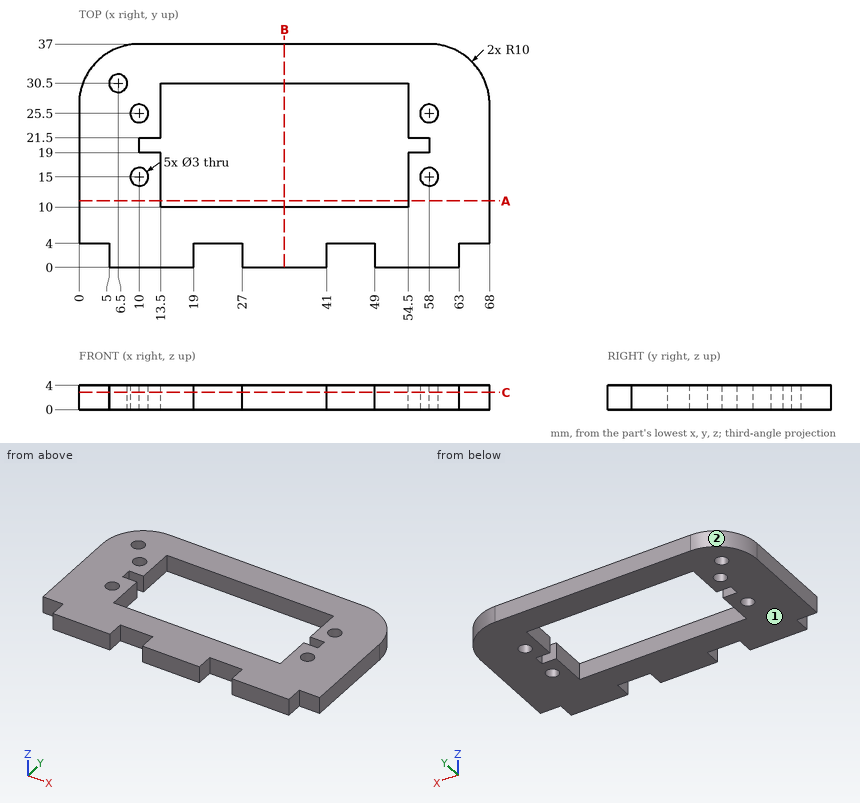
Geometry check sheet. Reference: drawing and pictorial views, mm from the part's lowest x, y, z. Give positions to 0.01 mm unless a question says otherwise; leave off trailing zeros. Loops run counter-clockwise (first coordinate to the right, second up) from the corner with the lowest first, then second, coordinate; pieces in that order, holes last. Notation, with made-up numbers: M 51.5,12 L 67.5,12 A15 cw 67.5,18 Z; hole C -28.75,83 d9. An arc over 180 degrees is marked long. Use a Markdown table: item, result. Add a question column.
Q1. Sectioned sample at B-B, the plane x = 34. Record the cut outline in (y, z).
Q2. Sectioned sample at A-A, the plane y = 11. Record the cut outline in (x, z).
Q3. Go/stop test with flat-tipped pins: pin 1 (1.2 mm diameter, centred on y = 1.5, z = 2, fed in from +X); pin 2 (1.2 mm diameter, centred on y = 2.5, z = 2, fed in from -X); pin 3 (1.2 mm diameter, centred on x = 66.5, z = 1.5, fed in from -Y); pin 4 (2.5 mm diameter, centred on x = 6.5, y = 30.5, fed in from +Z). Record where each tip stops, or that it passes through.
Q4. Sectioned sample at C-C, the plane z = 2.85. Give the number of separate pieces and of enclosed holes in the cut face, then the cut area to 3 significant figures.
Q5. Scan lines: line 1 along Y through (x, z) = (47, 1.45); line 2 along Y through (x, z) = (13, 0.95); line 3 along X through (y, z) = (20, 1.2). Record each from-to range of solid material in increasing order. Write a range as [from, to].
Q6. Mould release check, pull along X, two halves, no side actions. Record for the marked faces 1 and 2: pulls with the +X half, pulls with the -X half, needs draft (parallel to the pull), parting line crosses it, or undercut.
Verdict:
| question | item | result |
|---|---|---|
| 1 | outline | M 0,0 L 10,0 L 10,4 L 0,4 Z; M 30.5,0 L 37,0 L 37,4 L 30.5,4 Z |
| 2 | outline | M 0,0 L 13.5,0 L 13.5,4 L 0,4 Z; M 54.5,0 L 68,0 L 68,4 L 54.5,4 Z |
| 3 | pin 1 | x = 63 |
| 3 | pin 2 | x = 5 |
| 3 | pin 3 | y = 4 |
| 3 | pin 4 | through |
| 4 | separate pieces | 1 |
| 4 | enclosed holes | 6 |
| 4 | area | 1,480 mm^2 |
| 5 | line 1 | [4, 10], [30.5, 37] |
| 5 | line 2 | [0, 19], [21.5, 37] |
| 5 | line 3 | [0, 10], [58, 68] |
| 6 | face 1 | needs draft |
| 6 | face 2 | pulls with the -X half |
